```python
from build123d import *

# Parameters (mm, degrees)
F0_R     = 3.35
F1_DEPTH = 12
F3_DEPTH = 5
F5_DEPTH = 8
F6_W     = 100
F6_H     = 56
F7_DEPTH = 2
F8_R     = 5


with BuildPart() as f1:
    # F0 (on Front) → F1 (new body)
    with BuildSketch(Plane.XZ):
        Polygon((-65, 5), (-65, 0), (65, 0), (65, 5), (50, 5), (50, 61), (-50, 61), (-50, 5), align=None)
        with Locations((-38, 20.5)):
            Circle(F0_R, mode=Mode.SUBTRACT)
        with Locations((38, 20.5)):
            Circle(F0_R, mode=Mode.SUBTRACT)
        with Locations((-38, 45.5)):
            Circle(F0_R, mode=Mode.SUBTRACT)
        with Locations((38, 45.5)):
            Circle(F0_R, mode=Mode.SUBTRACT)
    extrude(amount=F1_DEPTH)

    # F2 (on face) → F3 (cut, through all)
    with BuildSketch(Plane(origin=(0, 0, 0), x_dir=(1, 0, 0), z_dir=(0, 0, -1))):
        with BuildLine():
            Line((-65, 2.65), (-63, 2.65))
            ThreePointArc((-63, 2.65), (-59.65, 6), (-63, 9.35))
            Line((-63, 9.35), (-65, 9.35))
            Line((-65, 9.35), (-65, 2.65))
        make_face()
        with BuildLine():
            Line((65, 9.35), (63, 9.35))
            ThreePointArc((63, 9.35), (59.65, 6), (63, 2.65))
            Line((63, 2.65), (65, 2.65))
            Line((65, 2.65), (65, 9.35))
        make_face()
    extrude(amount=-F3_DEPTH, mode=Mode.SUBTRACT)

    # F4 (on face) → F5 (cut)
    with BuildSketch(Plane(origin=(0, 0, 0), x_dir=(-1, 0, 0), z_dir=(0, 1, 0))):
        Polygon((35.113249, 25.5), (32.226497, 20.5), (35.113249, 15.5), (40.886751, 15.5), (43.773503, 20.5), (40.886751, 25.5), align=None)
        Polygon((-40.886751, 25.5), (-43.773503, 20.5), (-40.886751, 15.5), (-35.113249, 15.5), (-32.226497, 20.5), (-35.113249, 25.5), align=None)
        Polygon((35.113249, 50.5), (32.226497, 45.5), (35.113249, 40.5), (40.886751, 40.5), (43.773503, 45.5), (40.886751, 50.5), align=None)
        Polygon((-40.886751, 50.5), (-43.773503, 45.5), (-40.886751, 40.5), (-35.113249, 40.5), (-32.226497, 45.5), (-35.113249, 50.5), align=None)
    extrude(amount=-F5_DEPTH, mode=Mode.SUBTRACT)

    # F6 (on face) → F7 (cut)
    with BuildSketch(Plane(origin=(0, 0, 0), x_dir=(-1, 0, 0), z_dir=(0, 1, 0))):
        with Locations((0, 33)):
            Rectangle(F6_W, F6_H)
    extrude(amount=-F7_DEPTH, mode=Mode.SUBTRACT)

    # F8
    f8_edges = [f1.edges().sort_by_distance(p)[0] for p in [
        (-50, -7, 61),
        (50, -7, 61),
    ]]
    fillet(f8_edges, radius=F8_R)


solid = f1.part
```
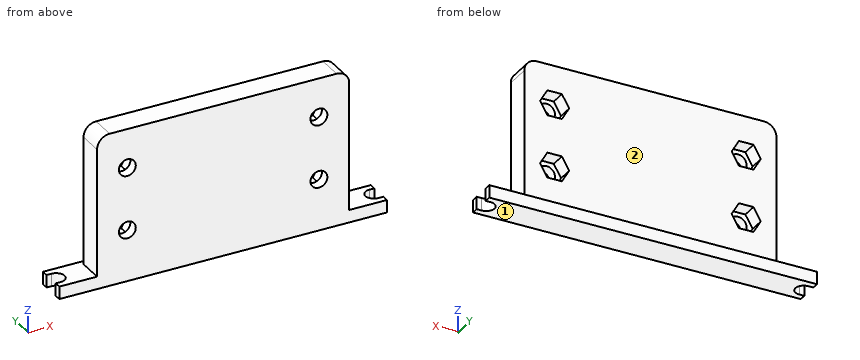
For this review, take the finished solid that the model builds, in its own axes (mm). Face numbers are marked on the shaded views. A direction names the side the tool comes from. Give positions to 0.01 mm unless a question says otherwise; leave off trailing zeros. Write each loop counter-clockwise with the first axis right and the second up, starting at its lowest first coordinate (ties: lowest second). Pieces come first, ordered by that corner, then holes. Notation, with made-up numbers: M -8.5,-22 L 40.5,-22 A20 ccw 40.5,12 Z; hole C -6.5,4 d2. An arc over 180 degrees is marked long. Answer as a JSON object with one key per item and string values. Group by question number.
Item 1: Tool access review of the marked faces 1 and 2: name each direction out of +Z, -Z, +X, -X, +Y, -Y from which nothing blocks a thin tool from reaching the whole face with its end or side.
Item 2: For probe 1 along Z at (x, y) = (38, -10.9); probe 2 along X at (y, z) = (-9.7, 45.5); probe 3 along Z at (x, y) = (41.5, -7.5), list the stretches that pass through material, from the lowest coordinate up. Write a range as [from, to].
Item 3: Consider section D-D on x = 53. Write out the cut boundary in (y, z).
Item 4: Consider section A-A on x = -38. Write out the cut boundary in (y, z), plus the area to 3 significant figures.
Item 5: Consider section B-B on x = -4. Write out the cut boundary in (y, z).
Item 6: Consider section C-C on z = 30. Write out the cut boundary in (x, y).
Item 7: For pin 1 Ø2 at (x, z) = (28.5, 11) entering from +Y; pin 2 Ø3 at (y, z) = (-10, 37) entering from -X; pin 3 Ø8.5 at (x, z) = (-38, 45.5) entering from +Y, all flat-tipped, find the tip position at first contact; note any pin that passes through.
Check result:
{
 "1": {"face 1": "-Z, +X, -X, +Y, -Y", "face 2": "+Z, +X, -X, +Y"},
 "2": {"probe 1": "z = [0, 17.15], [23.85, 42.15], [48.85, 61]", "probe 2": "x = [-50, -41.35], [-34.65, 34.65], [41.35, 50]", "probe 3": "z = [0, 16.56], [24.44, 41.56], [49.44, 61]"},
 "3": {"outline": "M -12,0 L 0,0 L 0,5 L -12,5 Z"},
 "4": {"outline": "M -12,0 L 0,0 L 0,5 L -2,5 L -2,15.5 L -8,15.5 L -8,17.15 L -12,17.15 Z; M -12,23.85 L -8,23.85 L -8,25.5 L -2,25.5 L -2,40.5 L -8,40.5 L -8,42.15 L -12,42.15 Z; M -12,48.85 L -8,48.85 L -8,50.5 L -2,50.5 L -2,61 L -12,61 Z", "area": "446 mm^2"},
 "5": {"outline": "M -12,0 L 0,0 L 0,5 L -2,5 L -2,61 L -12,61 Z"},
 "6": {"outline": "M -50,-12 L 50,-12 L 50,-2 L -50,-2 Z"},
 "7": {"pin 1": "stops at y = -2", "pin 2": "stops at x = -50", "pin 3": "stops at y = -8"}
}
